```python
from build123d import *

# Parameters (mm, degrees)
F0_W     = 97.109213
F0_H     = 76.168887
F1_DEPTH = 36.286205
F2_R     = 4.947674
F3_DEPTH = 51.584408
F4_W     = 35.460181
F4_H     = 26.693367
F5_DEPTH = 71.737379


with BuildPart() as f1:
    # F0 (on Front) → F1 (new body)
    with BuildSketch(Plane.XZ):
        with Locations((6.184138, -6.245349)):
            Rectangle(F0_W, F0_H)
    extrude(amount=F1_DEPTH)

    # F2 (on Front) → F3 (join)
    with BuildSketch(Plane.XZ):
        with Locations((34.461668, 17.535143)):
            Circle(F2_R)
    extrude(amount=F3_DEPTH)

    # F4 (on Front) → F5 (join)
    with BuildSketch(Plane.XZ):
        with Locations((10.323982, -41.378926)):
            Rectangle(F4_W, F4_H)
    extrude(amount=F5_DEPTH)


solid = f1.part
```
Work out the finished part from the listing and answer in its coordinate system (mm). A direction names the side the tool comes from. Give positions to 0.01 mm unless a question says otherwise; leave off trailing zeros. Loops run counter-clockwise (first coordinate to the right, second up) from the corner with the lowest first, then second, coordinate; pieces in that order, holes last. Notation, with made-up numbers: (66.25, 40.25) -> (124.25, 40.25) arc R22 ccw to (124.25, 46.25) -> close; hole circle Ø10 at (-30.5, 34.5). An arc over 180 degrees is marked (long way). Use CSV: the item, a comma, the result in double quotes.
1. The part is cut by section A-A (x = 10.5). Write down the section's boundary in (y, z), then the cut area to 3 significant figures.
Found:
outline,"(-71.74, -54.73) -> (0, -54.73) -> (0, 31.84) -> (-36.29, 31.84) -> (-36.29, -28.03) -> (-71.74, -28.03) -> close"
area,"4,090 mm^2"
2. The part is cut by section C-C (y = -43). Write down the section's boundary in (x, z), then the cut area to 3 significant figures.
Found:
outline,"(-7.41, -54.73) -> (28.05, -54.73) -> (28.05, -28.03) -> (-7.41, -28.03) -> close; circle Ø9.9 at (34.46, 17.54)"
area,"1,020 mm^2"
3. The part is cut by section B-B (y = -23). Write down the section's boundary in (x, z), then the cut area to 3 significant figures.
Found:
outline,"(-42.37, -44.33) -> (-7.41, -44.33) -> (-7.41, -54.73) -> (28.05, -54.73) -> (28.05, -44.33) -> (54.74, -44.33) -> (54.74, 31.84) -> (-42.37, 31.84) -> close"
area,"7,770 mm^2"
4. Straight lines are drawn through the part: line 1 (Y direction, x = -31.5, z = 26.5); line 2 (Z direction, x = -25, y = -21.5); line 3 (X direction, y = -62.5, z = -29). For each, find the intervals that lie inside material, in ascending order.
Found:
line 1,"-36.29 to 0"
line 2,"-44.33 to 31.84"
line 3,"-7.41 to 28.05"
5. The part is cut by section D-D (z = -10). Write down the section's boundary in (x, y).
Found:
outline,"(-42.37, -36.29) -> (54.74, -36.29) -> (54.74, 0) -> (-42.37, 0) -> close"
6. A tool of negligible diameter and unlimited length cuts with its end or side. For faces 1 (the flat face through (10, -54, -28.032)), 2 (the flat face through (41, -18, -44.33)), 3 (the cylindrical face through (30.54, -43.83, 14.52)), 4 (the flat face through (-25, -18, -44.33)), from which of +Z, -Z, +X, -X, +Y, -Y can it reach the whole face along a straight path? Write none if from no direction.
Found:
face 1,"+Z, +X, -X, -Y"
face 2,"-Z, +X, +Y, -Y"
face 3,"-Y"
face 4,"-Z, -X, +Y, -Y"
7. Flat-ended cylindrical pins translate along their axes: pin 1 Ø6 at (x, z) = (-10, 20) entering from -Y; pin 2 Ø3 at (x, z) = (33.5, 16) entering from -Y. Find the tip coordinate at first contact, or state that the pin passes through.
Found:
pin 1,"y = -36.29"
pin 2,"y = -51.58"
